Here's how the part is built. I have some questions about the finished solid (model axes, mm). Face numbers are marked on the shaded views. A direction names the side the tool comes from. Round coordinates to 2 decimals unless told otherwise and drop trailing zeros. Order: outer loops, then holes, each group sorted by start corner. A loop starts at its lowest first (then second) coordinate and runs counter-clockwise, first axis right, second up.
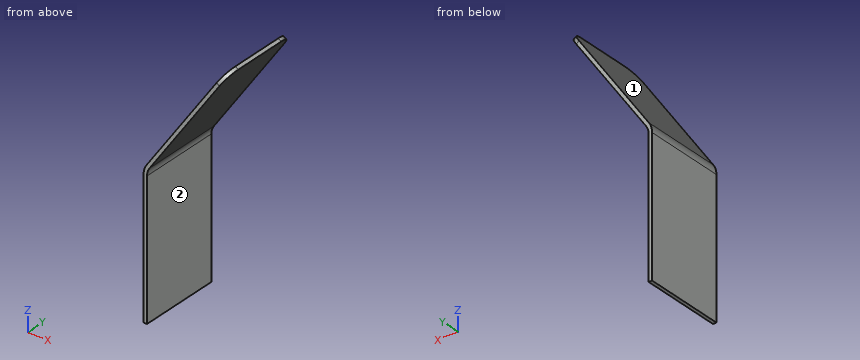
```python
from build123d import *

# Parameters (mm, degrees)
F1_DEPTH = 38.1
F2_R     = 6.35


with BuildPart() as f1:
    # F0 (on Front) → F1 (new body)
    with BuildSketch(Plane.XZ):
        with BuildLine():
            Line((0, -63.5), (0, -2.002147))
            ThreePointArc((0, -2.002147), (0.293897, -0.092665), (1.148385, 1.640063))
            Line((1.148385, 1.640063), (36.422104, 52.016155))
            Line((36.422104, 52.016155), (35.1217, 52.926707))
            Line((35.1217, 52.926707), (-0.152019, 2.550616))
            ThreePointArc((-0.152019, 2.550616), (-1.220128, 0.384705), (-1.5875, -2.002147))
            Line((-1.5875, -2.002147), (-1.5875, -63.5))
            Line((-1.5875, -63.5), (0, -63.5))
        make_face()
    extrude(amount=F1_DEPTH)

    # F2
    f2_edges = [f1.edges().sort_by_distance(p)[0] for p in [
        (35.771902, -38.1, 52.471431),
        (35.771902, 0, 52.471431),
    ]]
    fillet(f2_edges, radius=F2_R)


solid = f1.part
```
1. I need wall thicknesses on probe 1 along X at (y, z) = (-18, -39.5); probe 2 along Z at (x, y) = (17.5, -4); probe 3 along Z at (x, y) = (15, -34). Which ranges of each line are inside material? Lowest first, please.
Evaluation:
probe 1: x = -1.59 to 0
probe 2: z = 24.99 to 27.76
probe 3: z = 21.42 to 24.19
2. If we section it at C-C, the plane x = 22: Write out the boundary of the cut face in (y, z).
Evaluation:
outline: (-38.1, 31.42) - (0, 31.42) - (0, 34.19) - (-38.1, 34.19) - close
3. If we section it at B-B, the plane z = -20: Write out the boundary of the cut face in (x, y), and give its area (3 significant figures).
Evaluation:
outline: (-1.59, -38.1) - (0, -38.1) - (0, 0) - (-1.59, 0) - close
area: 60.5 mm2
4. On a 3-axis mill with a long thin cutter (end or side, diameter ignored), from which of +Z, -Z, +X, -X, +Y, -Y can I reach the whole of each face in a straight line? I mean the marked faces 1 and 2. Say none if no direction works.
Evaluation:
face 1: +Z, -X, +Y, -Y
face 2: -Z, +X, +Y, -Y
5. I'm going to push flat-ended pins straight in: P1, Ø19, axis at y = -12, z = -43, coming from the +X side; P2, Ø2, axis at x = 10, y = -6.5, coming from the -Z side; P3, Ø6, axis at x = 28, y = -32, coming from the -Z side. Where does each tip first touch, or does it pass through?
Evaluation:
P1: stops at x = 0
P2: stops at z = 12.85
P3: stops at z = 35.7
